Could you check a few things on this model? Use its own coordinates, in mm. A direction names the side the tool comes from. Round coordinates to 2 decimals unless told otherwise and drop trailing zeros. Loops run counter-clockwise (first coordinate to the right, second up) from the corner with the lowest first, then second, coordinate; pieces in that order, holes last. Notation, with made-up numbers: (5.5, 77.25) -> (34.5, 77.25) arc R16 cw to (34.5, 94.25) -> close; hole circle Ø8 at (18, -28.5). An arc over 180 degrees is marked (long way). One line per item, written item: value.
```python
from build123d import *

# Parameters (mm, degrees)
F_0000_CYLINDER_SKETCH_R     = 29
F_0000_CYLINDER_DEPTH        = 42.7
F_0000_CYLINDER_ROTATE_ANGLE = 90
F_0002_CYLINDER_SKETCH_R     = 26.8
F_0002_CYLINDER_DEPTH        = 39.7
F_0002_CYLINDER_ROTATE_ANGLE = 90
F_0005_CYLINDER_SKETCH_R     = 10
F_0005_CYLINDER_DEPTH        = 16.3
F_0005_CYLINDER_ROTATE_ANGLE = 90
F_0008_CYLINDER_SKETCH_R     = 3
F_0008_CYLINDER_DEPTH        = 20.9
F_0008_CYLINDER_ROTATE_ANGLE = 90
F_0011_CYLINDER_SKETCH_R     = 1.45
F_0011_CYLINDER_DEPTH        = 4.2
F_0011_CYLINDER_ROTATE_ANGLE = 90
F_0015_CYLINDER_SKETCH_R     = 1.45
F_0015_CYLINDER_DEPTH        = 4.2
F_0015_CYLINDER_ROTATE_ANGLE = 90
F_0019_CYLINDER_SKETCH_R     = 1.45
F_0019_CYLINDER_DEPTH        = 4.2
F_0019_CYLINDER_ROTATE_ANGLE = 90
F_0023_CYLINDER_SKETCH_R     = 1.45
F_0023_CYLINDER_DEPTH        = 4.2
F_0023_CYLINDER_ROTATE_ANGLE = 90
F_0027_BOX_SKETCH_W          = 31.1
F_0027_BOX_SKETCH_H          = 12
F_0027_BOX_DEPTH             = 28
F_0027_BOX_ROTATE_ANGLE      = 45
F_0031_CYLINDER_SKETCH_R     = 1.4
F_0031_CYLINDER_DEPTH        = 12.02
F_0031_CYLINDER_ROTATE_ANGLE = 90
F_0035_CYLINDER_SKETCH_R     = 1.4
F_0035_CYLINDER_DEPTH        = 12.02
F_0035_CYLINDER_ROTATE_ANGLE = 90
F_0039_CYLINDER_SKETCH_R     = 1.4
F_0039_CYLINDER_DEPTH        = 12.02
F_0039_CYLINDER_ROTATE_ANGLE = 90
F_0043_CYLINDER_SKETCH_R     = 1.4
F_0043_CYLINDER_DEPTH        = 12.02
F_0043_CYLINDER_ROTATE_ANGLE = 90
F_0047_CONE_ROTATE_ANGLE     = 120


with BuildPart() as part:
    # 0000_cylinder_Sketch → 0000_cylinder (new body)
    with BuildSketch(Plane.XY):
        with Locations(Location((0, 0, 0), (0, 0, 180))):
            Circle(F_0000_CYLINDER_SKETCH_R)
    extrude(amount=F_0000_CYLINDER_DEPTH)


with BuildPart() as part_1:
    # 0000_cylinder_Rotate: moved
    add(part.part.rotate(Axis((0, 0, 0), (0, 1, 0)), F_0000_CYLINDER_ROTATE_ANGLE))


with BuildPart() as part_2:
    # 0000_cylinder_Translate: moved
    add(part_1.part.moved(Location((-21.5, 0, 0))))


with BuildPart() as body_2:
    # 0002_cylinder_Sketch → 0002_cylinder (new body)
    with BuildSketch(Plane.XY):
        Circle(F_0002_CYLINDER_SKETCH_R)
    extrude(amount=F_0002_CYLINDER_DEPTH)


with BuildPart() as body_2_1:
    # 0002_cylinder_Rotate: moved
    add(body_2.part.rotate(Axis((0, 0, 0), (0, 1, 0)), F_0002_CYLINDER_ROTATE_ANGLE))


with BuildPart() as body_2_2:
    # 0002_cylinder_Translate: moved
    add(body_2_1.part.moved(Location((-22.5, 0, 0))))


with BuildPart() as part_3:
    add(part_2.part)

    # 0004_sub: cut body 2
    add(body_2_2.part, mode=Mode.SUBTRACT)


with BuildPart() as body_2_2_1:
    # 0005_cylinder_Sketch → 0005_cylinder (new body)
    with BuildSketch(Plane.XY):
        Circle(F_0005_CYLINDER_SKETCH_R)
    extrude(amount=F_0005_CYLINDER_DEPTH)


with BuildPart() as body_2_2_2:
    # 0005_cylinder_Rotate: moved
    add(body_2_2_1.part.rotate(Axis((0, 0, 0), (0, 1, 0)), F_0005_CYLINDER_ROTATE_ANGLE))


with BuildPart() as body_2_2_3:
    # 0005_cylinder_Translate: moved
    add(body_2_2_2.part.moved(Location((20.7, 0, 0))))


with BuildPart() as part_4:
    add(part_3.part)

    # 0007_add: union body 2 2
    add(body_2_2_3.part)


with BuildPart() as body_2_3:
    # 0008_cylinder_Sketch → 0008_cylinder (new body)
    with BuildSketch(Plane.XY):
        Circle(F_0008_CYLINDER_SKETCH_R)
    extrude(amount=F_0008_CYLINDER_DEPTH)


with BuildPart() as body_2_3_1:
    # 0008_cylinder_Rotate: moved
    add(body_2_3.part.rotate(Axis((0, 0, 0), (0, 1, 0)), F_0008_CYLINDER_ROTATE_ANGLE))


with BuildPart() as body_2_3_2:
    # 0008_cylinder_Translate: moved
    add(body_2_3_1.part.moved(Location((17.1, 0, 0))))


with BuildPart() as part_5:
    add(part_4.part)

    # 0010_sub: cut body 2 3
    add(body_2_3_2.part, mode=Mode.SUBTRACT)


with BuildPart() as body_2_4:
    # 0011_cylinder_Sketch → 0011_cylinder (new body)
    with BuildSketch(Plane.XY):
        Circle(F_0011_CYLINDER_SKETCH_R)
    extrude(amount=F_0011_CYLINDER_DEPTH)


with BuildPart() as body_2_4_1:
    # 0011_cylinder_Rotate: moved
    add(body_2_4.part.rotate(Axis((0, 0, 0), (0, 1, 0)), F_0011_CYLINDER_ROTATE_ANGLE))


with BuildPart() as body_2_4_2:
    # 0011_cylinder_Translate: moved
    add(body_2_4_1.part.moved(Location((17.1, 23.5, 0))))


with BuildPart() as part_6:
    add(part_5.part)

    # 0014_sub: cut body 2 4
    add(body_2_4_2.part, mode=Mode.SUBTRACT)


with BuildPart() as body_2_5:
    # 0015_cylinder_Sketch → 0015_cylinder (new body)
    with BuildSketch(Plane.XY):
        Circle(F_0015_CYLINDER_SKETCH_R)
    extrude(amount=F_0015_CYLINDER_DEPTH)


with BuildPart() as body_2_5_1:
    # 0015_cylinder_Rotate: moved
    add(body_2_5.part.rotate(Axis((0, 0, 0), (0, 1, 0)), F_0015_CYLINDER_ROTATE_ANGLE))


with BuildPart() as body_2_5_2:
    # 0015_cylinder_Translate: moved
    add(body_2_5_1.part.moved(Location((17.1, 0, 23.5))))


with BuildPart() as part_7:
    add(part_6.part)

    # 0018_sub: cut body 2 5
    add(body_2_5_2.part, mode=Mode.SUBTRACT)


with BuildPart() as body_2_6:
    # 0019_cylinder_Sketch → 0019_cylinder (new body)
    with BuildSketch(Plane.XY):
        Circle(F_0019_CYLINDER_SKETCH_R)
    extrude(amount=F_0019_CYLINDER_DEPTH)


with BuildPart() as body_2_6_1:
    # 0019_cylinder_Rotate: moved
    add(body_2_6.part.rotate(Axis((0, 0, 0), (0, 1, 0)), F_0019_CYLINDER_ROTATE_ANGLE))


with BuildPart() as body_2_6_2:
    # 0019_cylinder_Translate: moved
    add(body_2_6_1.part.moved(Location((17.1, -23.5, 0))))


with BuildPart() as part_8:
    add(part_7.part)

    # 0022_sub: cut body 2 6
    add(body_2_6_2.part, mode=Mode.SUBTRACT)


with BuildPart() as body_2_7:
    # 0023_cylinder_Sketch → 0023_cylinder (new body)
    with BuildSketch(Plane.XY):
        Circle(F_0023_CYLINDER_SKETCH_R)
    extrude(amount=F_0023_CYLINDER_DEPTH)


with BuildPart() as body_2_7_1:
    # 0023_cylinder_Rotate: moved
    add(body_2_7.part.rotate(Axis((0, 0, 0), (0, 1, 0)), F_0023_CYLINDER_ROTATE_ANGLE))


with BuildPart() as body_2_7_2:
    # 0023_cylinder_Translate: moved
    add(body_2_7_1.part.moved(Location((17.1, 0, -23.5))))


with BuildPart() as part_9:
    add(part_8.part)

    # 0026_sub: cut body 2 7
    add(body_2_7_2.part, mode=Mode.SUBTRACT)


with BuildPart() as body_2_8:
    # 0027_box_Sketch → 0027_box (new body)
    with BuildSketch(Plane.XY):
        with Locations((15.55, 6)):
            Rectangle(F_0027_BOX_SKETCH_W, F_0027_BOX_SKETCH_H)
    extrude(amount=F_0027_BOX_DEPTH)


with BuildPart() as body_2_8_1:
    # 0027_box_Rotate: moved
    add(body_2_8.part.rotate(Axis((0, 0, 0), (-1, 0, 0)), F_0027_BOX_ROTATE_ANGLE))


with BuildPart() as body_2_8_2:
    # 0027_box_Translate: moved
    add(body_2_8_1.part.moved(Location((6, 0.707106781, 9.192388155))))


with BuildPart() as part_10:
    add(part_9.part)

    # 0030_sub: cut body 2 8
    add(body_2_8_2.part, mode=Mode.SUBTRACT)


with BuildPart() as body_2_9:
    # 0031_cylinder_Sketch → 0031_cylinder (new body)
    with BuildSketch(Plane.XY):
        with Locations(Location((0, 0, 0), (0, 0, 180))):
            Circle(F_0031_CYLINDER_SKETCH_R)
    extrude(amount=F_0031_CYLINDER_DEPTH)


with BuildPart() as body_2_9_1:
    # 0031_cylinder_Rotate: moved
    add(body_2_9.part.rotate(Axis((0, 0, 0), (0, 1, 0)), F_0031_CYLINDER_ROTATE_ANGLE))


with BuildPart() as body_2_9_2:
    # 0031_cylinder_Translate: moved
    add(body_2_9_1.part.moved(Location((24.99, 6.5, 0))))


with BuildPart() as part_11:
    add(part_10.part)

    # 0034_sub: cut body 2 9
    add(body_2_9_2.part, mode=Mode.SUBTRACT)


with BuildPart() as body_2_10:
    # 0035_cylinder_Sketch → 0035_cylinder (new body)
    with BuildSketch(Plane.XY):
        with Locations(Location((0, 0, 0), (0, 0, 180))):
            Circle(F_0035_CYLINDER_SKETCH_R)
    extrude(amount=F_0035_CYLINDER_DEPTH)


with BuildPart() as body_2_10_1:
    # 0035_cylinder_Rotate: moved
    add(body_2_10.part.rotate(Axis((0, 0, 0), (0, 1, 0)), F_0035_CYLINDER_ROTATE_ANGLE))


with BuildPart() as body_2_10_2:
    # 0035_cylinder_Translate: moved
    add(body_2_10_1.part.moved(Location((24.99, 0, 6.5))))


with BuildPart() as part_12:
    add(part_11.part)

    # 0038_sub: cut body 2 10
    add(body_2_10_2.part, mode=Mode.SUBTRACT)


with BuildPart() as body_2_11:
    # 0039_cylinder_Sketch → 0039_cylinder (new body)
    with BuildSketch(Plane.XY):
        with Locations(Location((0, 0, 0), (0, 0, 180))):
            Circle(F_0039_CYLINDER_SKETCH_R)
    extrude(amount=F_0039_CYLINDER_DEPTH)


with BuildPart() as body_2_11_1:
    # 0039_cylinder_Rotate: moved
    add(body_2_11.part.rotate(Axis((0, 0, 0), (0, 1, 0)), F_0039_CYLINDER_ROTATE_ANGLE))


with BuildPart() as body_2_11_2:
    # 0039_cylinder_Translate: moved
    add(body_2_11_1.part.moved(Location((24.99, -6.5, 0))))


with BuildPart() as part_13:
    add(part_12.part)

    # 0042_sub: cut body 2 11
    add(body_2_11_2.part, mode=Mode.SUBTRACT)


with BuildPart() as body_2_12:
    # 0043_cylinder_Sketch → 0043_cylinder (new body)
    with BuildSketch(Plane.XY):
        with Locations(Location((0, 0, 0), (0, 0, 180))):
            Circle(F_0043_CYLINDER_SKETCH_R)
    extrude(amount=F_0043_CYLINDER_DEPTH)


with BuildPart() as body_2_12_1:
    # 0043_cylinder_Rotate: moved
    add(body_2_12.part.rotate(Axis((0, 0, 0), (0, 1, 0)), F_0043_CYLINDER_ROTATE_ANGLE))


with BuildPart() as body_2_12_2:
    # 0043_cylinder_Translate: moved
    add(body_2_12_1.part.moved(Location((24.99, 0, -6.5))))


with BuildPart() as part_14:
    add(part_13.part)

    # 0046_sub: cut body 2 12
    add(body_2_12_2.part, mode=Mode.SUBTRACT)


with BuildPart() as body_2_13:
    # 0047_cone_Sketch → 0047_cone (revolve)
    with BuildSketch(Plane.XY, mode=Mode.PRIVATE) as f_0047_cone_sk:
        Polygon((0, 0), (26.8, 0), (27.3, 0.51), (0, 0.51), align=None)
    revolve(f_0047_cone_sk.sketch.rotate(Axis((0, -100, 0), (0, 1, 0)), 90), axis=Axis((0, -100, 0), (0, 1, 0)))


with BuildPart() as body_2_13_1:
    # 0047_cone_Rotate: moved
    add(body_2_13.part.rotate(Axis((0, 0, 0), (0.5773502691896258, -0.5773502691896257, -0.5773502691896257)), F_0047_CONE_ROTATE_ANGLE))


with BuildPart() as body_2_13_2:
    # 0047_cone_Translate: moved
    add(body_2_13_1.part.moved(Location((-21, 0, 0))))


with BuildPart() as part_15:
    add(part_14.part)

    # 0050_sub: cut body 2 13
    add(body_2_13_2.part, mode=Mode.SUBTRACT)


solid = part_15.part
```
(1) On a 3-axis mill with a long thin cutter (end or side, diameter ignored), from which of +Z, -Z, +X, -X, +Y, -Y can I reach the whole of each face in a straight line? I mean faces 1 (the face through (-2.42, -10.26, -24.76)), 2 (the face through (28.989, -7.314, -6.819)), 3 (the face through (19.17, 0.44, 22.12)). Say none if no direction works.
Results below:
face 1: -X
face 2: +X
face 3: +X, -X
(2) For pin 1 Ø4 at (y, z) = (23.5, 0) entering from -X; pin 2 Ø1 at (x, z) = (-7, 2.5) entering from -Y; pin 3 Ø2 at (x, y) = (-3, 18) entering from +Z, each with a flat end and sliding along its axis, tell me the tip position at first contact or that it passes through.
Results below:
pin 1: stops at x = 17.2
pin 2: stops at y = -28.93
pin 3: stops at z = 23.49
(3) We'd pull the mould along Z, two halves only. Please class faces 4 (the face through (27, 0, 3)), 5 (the face through (-21.5, 26, 8)), 6 (the face through (-0.45, 25.73, 13.38)): +Z half, -Z half, draft (parallel to the pull), parting line (faces both ways), or undercut.
Results below:
face 4: undercut
face 5: draft
face 6: parting line
(4) Please list where these lines run through material, in increasing order: L1, parallel to Y at x = 30, z = 0; L2, parallel to Y at x = 24, z = 1; L3, parallel to Y at x = -12, z = 0.
Results below:
L1: y = -10 to -7.9, -5.1 to -3, 3 to 5.1, 7.9 to 10
L2: y = -9.95 to -2.83, 2.83 to 8.9, 9.49 to 9.95
L3: y = -29 to -26.8, 26.8 to 29
(5) Imagine slicing it at C-C on z = -11.5. Write out the boundary of the cut face in (x, y).
Results below:
outline: (-21.5, -26.62) -> (21.2, -26.62) -> (21.2, 26.62) -> (-21.5, 26.62) -> (-21.5, 24.21) -> (17.2, 24.21) -> (17.2, -24.21) -> (-21.5, -24.21) -> close
(6) Imagine slicing it at A-A on z = -23.5. Write out the boundary of the cut face in (x, y).
Results below:
outline: (-21.5, -16.99) -> (21.2, -16.99) -> (21.2, -1.45) -> (17.2, -1.45) -> (17.2, -12.88) -> (-21.5, -12.88) -> close; (-21.5, 12.88) -> (17.2, 12.88) -> (17.2, 1.45) -> (21.2, 1.45) -> (21.2, 16.99) -> (-21.5, 16.99) -> close
(7) Imagine slicing it at D-D on x = -5. Write out the boundary of the cut face in (y, z), then the cut area to 3 significant figures.
Results below:
outline: circle Ø58 at (0, 0); hole circle Ø53.6 at (0, 0)
area: 386 mm²
(8) Imagine slicing it at B-B on y = -6.5. Write out the boundary of the cut face in (x, z).
Results below:
outline: (-21.5, -28.26) -> (21.2, -28.26) -> (21.2, -7.6) -> (37, -7.6) -> (37, -1.4) -> (24.99, -1.4) -> (24.99, 1.4) -> (37, 1.4) -> (37, 7.6) -> (21.2, 7.6) -> (21.2, 28.26) -> (-21.5, 28.26) -> (-21.5, 26) -> (17.2, 26) -> (17.2, -26) -> (-21.5, -26) -> close
